from build123d import *

# Parameters (mm, degrees)
F1_DEPTH  = 3.75
F2_W      = 3.75
F2_H      = 50
F3_DEPTH  = 3.75
F4_W      = 20
F4_H      = 3.75
F5_DEPTH  = 1.25
F7_D      = 6
F7_DEPTH  = 4
F7_TIP    = 1.8025818571
F8_W      = 30
F8_H      = 1.25
F9_DEPTH  = 3.75
F10_W     = 3.75
F10_H     = 50
F11_DEPTH = 3.75


# Not quite as in the source:
# - a feature names something its author has since deleted; it is built from what else it names


with BuildPart() as f1:
    # F0 (on Front) → F1 (new body)
    with BuildSketch(Plane.XZ):
        Polygon((50, -7.5), (50, 0), (150, 0), (150, -7.5), (200, -7.5), (200, 0), (300, 0), (300, -7.5), (350, -7.5), (350, 0), (350, 200), (0, 200), (-50, 200), (-50, 0), (0, 0), (0, -7.5), align=None)
    extrude(amount=F1_DEPTH)

    # F2 (on face) → F3 (cut)
    with BuildSketch(Plane.XZ.offset(3.75)):
        with Locations((325, 150)):
            Rectangle(F2_W, F2_H)
        with Locations((325, 67.5)):
            Rectangle(F2_W, F2_H)
    extrude(amount=-F3_DEPTH, mode=Mode.SUBTRACT)

    # F4 (on face) → F5 (join)
    with BuildSketch(Plane.XY.offset(200)):
        with Locations((80, -1.875)):
            Rectangle(F4_W, F4_H)
        with Locations((30, -1.875)):
            Rectangle(F4_W, F4_H)
        with Locations((-20, -1.875)):
            Rectangle(F4_W, F4_H)
    extrude(amount=F5_DEPTH)

    # F7
    with Locations(Plane(origin=(0, 0, 0), x_dir=(-1, 0, 0), z_dir=(0, 1, 0))):
        with Locations((-80, 91.25), (-80, 191.25), (-30, 91.25), (20, 91.25), (20, 191.25), (-30, 191.25)):
            Hole(F7_D / 2, depth=F7_DEPTH)
            with Locations((0, 0, -(F7_DEPTH + F7_TIP / 2))):  # 118° drill point
                Cone(0, F7_D / 2, F7_TIP, mode=Mode.SUBTRACT)

    # F8 (on face) → F9 (join)
    with BuildSketch(Plane(origin=(0, 0, 0), x_dir=(-1, 0, 0), z_dir=(0, 1, 0))):
        with Locations((-55, 200.625)):
            Rectangle(F8_W, F8_H)
        Polygon((30, 201.25), (30, 200), (50, 200), align=None)
        Polygon((-90, 200), (-90, 201.25), (-110, 200), align=None)
        Polygon((10, 201.25), (-5, 200), (10, 200), align=None)
        Polygon((-8.75, 200), (-20, 201.25), (-20, 200), align=None)
    extrude(amount=-F9_DEPTH)

    # F10 (on face) → F11 (cut)
    with BuildSketch(Plane(origin=(0, 0, 0), x_dir=(-1, 0, 0), z_dir=(0, 1, 0))):
        with Locations((-6.875, 150)):
            Rectangle(F10_W, F10_H)
        with Locations((-6.875, 67)):
            Rectangle(F10_W, F10_H)
    extrude(amount=-F11_DEPTH, mode=Mode.SUBTRACT)


solid = f1.part
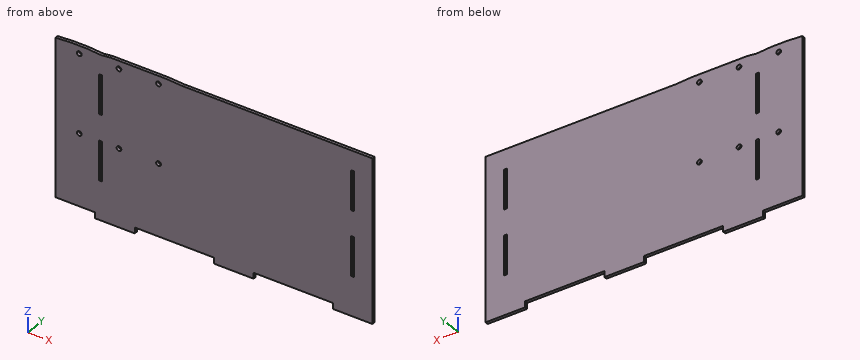
Source: CAD feature listing. Evaluate the final solid. Frame: model axes, mm. Give positions to 0.01 mm unless a question says otherwise; leave off trailing zeros. Order: outer loops, then holes, each group sorted by start corner. A loop starts at its lowest first (then second) coordinate and runs counter-clockwise, first axis right, second up. Notation, with made-up numbers: (4.25, 64.25) -> (11.25, 64.25) arc R27 cw to (11.25, 92.25) -> close; hole circle Ø11 at (33.5, 31). An arc over 180 degrees is marked (long way). Use a Markdown table: item, result.
1) Section query A-A, the plane z = 73.5. Return the cut outline in (x, y) (3 decimals).
Answer list:
| item | result |
|---|---|
| outline | (-50, -3.75) -> (5, -3.75) -> (5, 0) -> (-50, 0) -> close; (8.75, -3.75) -> (323.125, -3.75) -> (323.125, 0) -> (8.75, 0) -> close; (326.875, -3.75) -> (350, -3.75) -> (350, 0) -> (326.875, 0) -> close |
2) Contact query for flat-ended pins moving along their axis: P1, Ø3.5, axis at x = 80, z = 91.25, coming from the -Y side; P2, Ø1.9, axis at x = 7.5, y = -1, coming from the +Z side; P3, Ø1.1, axis at y = -1.5, z = -5.5, coming from the -X side. Output: stop coordinate, or through.
Answer list:
| item | result |
|---|---|
| P1 | through |
| P2 | z = 200 |
| P3 | x = 0 |
3) Section query B-B, the plane y = -2.3. Count the separate pieces of the cut face and the enclosed holes in it, then the cut area to 3 significant figures.
Answer list:
| item | result |
|---|---|
| separate pieces | 1 |
| enclosed holes | 10 |
| area | 80,400 mm² |
4) Ray query, line 1 along X through (y, z) = (-0.35, 55) (3 decimals); line 2 along X through (y, z) = (-1.4, 191.25); line 3 along Z through (x, y) = (80, -1.75). Return the intervals inside material, ascending. Write a range as [from, to].
Answer list:
| item | result |
|---|---|
| line 1 | [-50, 5], [8.75, 323.125], [326.875, 350] |
| line 2 | [-50, -23], [-17, 27], [33, 77], [83, 350] |
| line 3 | [0, 88.25], [94.25, 188.25], [194.25, 201.25] |
